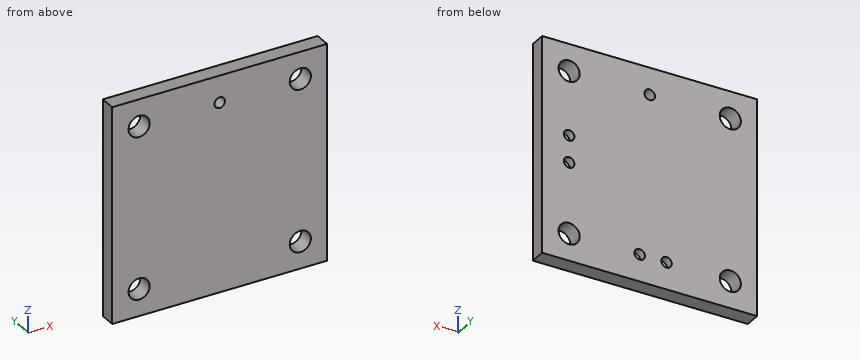
```python
from build123d import *

# Parameters (mm, degrees)
SKETCH1_W           = 20.32
SKETCH1_H           = 20.32
SKETCH1_R           = 1
SKETCH1_R_2         = 0.5
BOSS_EXTRUDE1_DEPTH = 1.5
CUT_EXTRUDE1_START  = 1.5
SKETCH1_3_R         = 0.5
CUT_EXTRUDE1_DEPTH  = 0.762


with BuildPart() as part:
    # Sketch1 → Boss-Extrude1 (new body)
    with BuildSketch(Plane(origin=(0, 0, 0), x_dir=(1, 0, 0), z_dir=(0, 1, 0))):
        with Locations((10.16, 10.16)):
            Rectangle(SKETCH1_W, SKETCH1_H)
        with Locations(Location((2.54, 2.54, 0), (0, 0, 270))):  # turned: the seam where the file's is
            Circle(SKETCH1_R, mode=Mode.SUBTRACT)
        with Locations(Location((17.78, 2.54, 0), (0, 0, 270))):  # turned: the seam where the file's is
            Circle(SKETCH1_R, mode=Mode.SUBTRACT)
        with Locations(Location((17.78, 17.78, 0), (0, 0, 270))):  # turned: the seam where the file's is
            Circle(SKETCH1_R, mode=Mode.SUBTRACT)
        with Locations(Location((2.54, 17.78, 0), (0, 0, 270))):  # turned: the seam where the file's is
            Circle(SKETCH1_R, mode=Mode.SUBTRACT)
        with Locations(Location((10.16, 2.54, 0), (0, 0, 270))):  # turned: the seam where the file's is
            Circle(SKETCH1_R_2, mode=Mode.SUBTRACT)
    extrude(amount=BOSS_EXTRUDE1_DEPTH)

    # Sketch1_3 → Cut-Extrude1 (cut)
    with BuildSketch(Plane(origin=(0, 0, 0), x_dir=(1, 0, 0), z_dir=(0, 1, 0)).offset(CUT_EXTRUDE1_START)):
        with Locations(Location((17.78, 11.11, 0), (0, 0, 270))):  # turned: the seam where the file's is
            Circle(SKETCH1_3_R)
        with Locations(Location((17.78, 8.57, 0), (0, 0, 270))):  # turned: the seam where the file's is
            Circle(SKETCH1_3_R)
        with Locations(Location((11.109999878, 17.78, 0), (0, 0, 90))):  # turned: the seam where the file's is
            Circle(SKETCH1_3_R)
        with Locations(Location((8.569999878, 17.78, 0), (0, 0, 270))):  # turned: the seam where the file's is
            Circle(SKETCH1_3_R)
    extrude(amount=-CUT_EXTRUDE1_DEPTH, mode=Mode.SUBTRACT)


solid = part.part
```
Geometry: final body of the model. Coordinates: model frame, mm. Coordinates: 2 decimals unless noted, no trailing zeros. Order: outer loops, then holes, each group sorted by start corner. A loop starts at its lowest first (then second) coordinate and runs counter-clockwise, first axis right, second up. Notation, with made-up numbers: (-23.5, 42.25) - (16.5, 42.25) arc R26 ccw to (16.5, 78.25) - close; hole circle Ø3 at (20, 46.5). An arc over 180 degrees is marked (long way). Write each question's results on one line, items separated by ' | '.
(1) Section query A-A, the plane z = -17.78. Return the cut outline in (x, y), plus the area to 3 significant figures.
Values found:
outline: (0, 0) - (1.54, 0) - (1.54, 1.5) - (0, 1.5) - close; (3.54, 0) - (16.78, 0) - (16.78, 1.5) - (11.61, 1.5) - (11.61, 0.74) - (10.61, 0.74) - (10.61, 1.5) - (9.07, 1.5) - (9.07, 0.74) - (8.07, 0.74) - (8.07, 1.5) - (3.54, 1.5) - close; (18.78, 0) - (20.32, 0) - (20.32, 1.5) - (18.78, 1.5) - close | area: 23.0 mm²
(2) Section query D-D, the plane z = -2.54. Return the cut outline in (x, y), plus the area to 3 significant figures.
Values found:
outline: (0, 0) - (1.54, 0) - (1.54, 1.5) - (0, 1.5) - close; (3.54, 0) - (9.66, 0) - (9.66, 1.5) - (3.54, 1.5) - close; (10.66, 0) - (16.78, 0) - (16.78, 1.5) - (10.66, 1.5) - close; (18.78, 0) - (20.32, 0) - (20.32, 1.5) - (18.78, 1.5) - close | area: 23.0 mm²
(3) Line query: line 1 (X direction, y = 0.8, z = -2.5); line 2 (Z direction, x = 8.57, y = 1.05); line 3 (Z direction, x = 10, y = 0.9). Output: solid intervals per line, ascending. Write a range as [from, to].
Values found:
line 1: x = [0, 1.54], [3.54, 9.66], [10.66, 16.78], [18.78, 20.32] | line 2: z = [-20.32, -18.28], [-17.28, 0] | line 3: z = [-20.32, -3.01], [-2.07, 0]
(4) Section query B-B, the plane y = 1.2. Count the separate pieces of the cut face and the enclosed holes in it, plus the area to 3 significant figures.
Values found:
separate pieces: 1 | enclosed holes: 9 | area: 396 mm²
(5) Section query C-C, the plane x = 11.11. Return the cut outline in (y, z).
Values found:
outline: (0, -20.32) - (1.5, -20.32) - (1.5, -18.28) - (0.74, -18.28) - (0.74, -17.28) - (1.5, -17.28) - (1.5, 0) - (0, 0) - close
